Could you check a few things on this model? Use its own coordinates, in mm. A direction names the side the tool comes from. Coordinates: 2 decimals unless noted, no trailing zeros. Use CSV: the item, a comma, the result in double quotes.
from build123d import *

# Parameters (mm, degrees)
SKETCH1_R           = 14
BOSS_EXTRUDE1_DEPTH = 2
SKETCH2_R           = 1.12
BOSS_EXTRUDE2_DEPTH = 10
SKETCH3_R           = 14
SKETCH3_R_2         = 11.76
BOSS_EXTRUDE3_DEPTH = 1
CHAMFER1_SIZE       = 0.5
SKETCH5_R           = 7
BOSS_EXTRUDE4_DEPTH = 2


with BuildPart() as part:
    # Sketch1 → Boss-Extrude1 (new body)
    with BuildSketch(Plane(origin=(0, 0, 0), x_dir=(1, 0, 0), z_dir=(0, 1, 0))):
        with Locations(Location((0, 0, 0), (0, 0, 270))):
            Circle(SKETCH1_R)
        Polygon((5, 0), (2.5, 4.330127019), (-2.5, 4.330127019), (-5, 0), (-2.5, -4.330127019), (2.5, -4.330127019), align=None, mode=Mode.SUBTRACT)
    extrude(amount=BOSS_EXTRUDE1_DEPTH)

    # Sketch2 → Boss-Extrude2 (add)
    with BuildSketch(Plane(origin=(0, 2, 0), x_dir=(1, 0, 0), z_dir=(0, 1, 0))):
        with BuildLine():
            ThreePointArc((0, 14), (-1.12, 12.88), (0, 11.76))
            Line((0, 11.76), (0, 14))
        make_face()
        with BuildLine():
            Line((0, 14), (0, 11.76))
            ThreePointArc((0, 11.76), (0.791959595, 12.088040405), (1.12, 12.88))
            ThreePointArc((1.12, 12.88), (0.791959595, 13.671959595), (0, 14))
        make_face()
        with Locations(Location((4.405219446, 12.103240956, 0), (0, 0, 69.999194591))):
            Circle(SKETCH2_R)
        with Locations(Location((8.279104413, 9.866652427, 0), (0, 0, 49.999187687))):
            Circle(SKETCH2_R)
        with Locations(Location((11.154407201, 6.44, 0), (0, 0, 29.999182162))):
            Circle(SKETCH2_R)
        with Locations(Location((12.684323859, 2.236588528, 0), (0, 0, 9.999177247))):
            Circle(SKETCH2_R)
        with Locations(Location((12.684323859, -2.236588528, 0), (0, 0, 349.999173281))):
            Circle(SKETCH2_R)
        with Locations(Location((11.154407201, -6.44, 0), (0, 0, 329.99917002))):
            Circle(SKETCH2_R)
        with Locations(Location((8.279104413, -9.866652427, 0), (0, 0, 309.999169093))):
            Circle(SKETCH2_R)
        with Locations(Location((4.405219446, -12.103240956, 0), (0, 0, 289.999169998))):
            Circle(SKETCH2_R)
        with Locations(Location((-4.405219446, -12.103240956, 0), (0, 0, 249.999176515))):
            Circle(SKETCH2_R)
        with Locations(Location((-8.279104413, -9.866652427, 0), (0, 0, 229.999182687))):
            Circle(SKETCH2_R)
        with Locations(Location((-11.154407201, -6.44, 0), (0, 0, 209.999188831))):
            Circle(SKETCH2_R)
        with Locations(Location((-12.684323859, -2.236588528, 0), (0, 0, 189.999194613))):
            Circle(SKETCH2_R)
        with Locations(Location((-12.684323859, 2.236588528, 0), (0, 0, 169.999199466))):
            Circle(SKETCH2_R)
        with Locations(Location((-11.154407201, 6.44, 0), (0, 0, 149.999202654))):
            Circle(SKETCH2_R)
        with Locations(Location((-8.279104413, 9.866652427, 0), (0, 0, 129.999204018))):
            Circle(SKETCH2_R)
        with Locations(Location((-4.405219446, 12.103240956, 0), (0, 0, 109.99920326))):
            Circle(SKETCH2_R)
        with Locations(Location((0, -12.88, 0), (0, 0, 269.999172475))):
            Circle(SKETCH2_R)
    extrude(amount=BOSS_EXTRUDE2_DEPTH)

    # Sketch3 → Boss-Extrude3 (add)
    with BuildSketch(Plane(origin=(0, 12, 0), x_dir=(1, 0, 0), z_dir=(0, 1, 0))):
        with Locations(Location((0, 0, 0), (0, 0, 90.000063859))):
            Circle(SKETCH3_R)
        with Locations(Location((0, 0, 0), (0, 0, 270))):
            Circle(SKETCH3_R_2, mode=Mode.SUBTRACT)
    extrude(amount=BOSS_EXTRUDE3_DEPTH)

    # Chamfer1
    chamfer1_edges = [part.edges().sort_by_distance(p)[0] for p in [
        (0, 0, -4.330127019),
        (-3.75, 0, -2.165063509),
        (-3.75, 0, 2.165063509),
        (0, 0, 4.330127019),
        (0, 0, -14),
        (3.75, 0, 2.165063509),
        (3.75, 0, -2.165063509),
    ]]
    chamfer(chamfer1_edges, length=CHAMFER1_SIZE)

    # Sketch5 → Boss-Extrude4 (add)
    with BuildSketch(Plane(origin=(0, 2, 0), x_dir=(1, 0, 0), z_dir=(0, 1, 0))):
        with Locations(Location((0, 0, 0), (0, 0, 270))):
            Circle(SKETCH5_R)
        Polygon((5, 0), (2.5, 4.330127019), (-2.5, 4.330127019), (-5, 0), (-2.5, -4.330127019), (2.5, -4.330127019), align=None, mode=Mode.SUBTRACT)
    extrude(amount=BOSS_EXTRUDE4_DEPTH)


solid = part.part
(1) Will these pins go through, and if not, where does the flat tip stop? pin 1 (3 mm diameter, centred on x = -8, y = 2.5, fed in from +Z); pin 2 (2 mm diameter, centred on y = 5.5, z = -1, fed in from -X); pin 3 (4 mm diameter, centred on x = -3, z = -1, fed in from +Y).
Computed:
pin 1,"stops at z = 12.35"
pin 2,"stops at x = -13.78"
pin 3,"stops at y = 4"
(2) Which directions (+Z, -Z, +X, -X, +Y, -Y) give clear straight access to the entire face, cutting with the end or side of a thin tool? Please do faces 1 (the face through (-6.834, 2.986, -1.517)), 2 (the face through (3.73, 2.23, 2.2)), 3 (the face through (-3.989, 0.247, 2.258)), 4 (the face through (-3.65, 6.93, -12.93)).
Computed:
face 1,"+Y"
face 2,"+Y, -Y"
face 3,"-Y"
face 4,"none"
(3) Please list where these lines run through material, in increasing order: line 1 (X direction, y = 12.4, z = 0); line 2 (X direction, y = 2.25, z = 1.25).
Computed:
line 1,"x = -14 to -11.76, 11.76 to 14"
line 2,"x = -13.21 to -12.15, -6.89 to -4.28, 4.28 to 6.89, 12.15 to 13.21"
(4) Suppose I cut it at A-A (y = 3). State how many separate pieces and enclosed holes the cut face has, plus the area to 3 significant figures.
Computed:
separate pieces,"19"
enclosed holes,"1"
area,"160 mm²"
